```python
from build123d import *

# Parameters (mm, degrees)
F0_R      = 10.5
F0_R_2    = 9.9
F1_DEPTH  = 1.7
F2_DEPTH  = 2.8
F3_R      = 10.5
F4_DEPTH  = 1.7
F5_R      = 11
F6_DEPTH  = 8
F7_SIZE2  = 4
F7_SIZE   = 3
F8_R      = 8
F9_DEPTH  = 5
F11_D     = 18
F11_DEPTH = 10
F11_TIP   = 5.4077455712
F13_D     = 12
F14_R     = 1


with BuildPart() as f1:
    # F0 (on Top) → F1 (new body)
    with BuildSketch(Plane.XY):
        Circle(F0_R)
        Circle(F0_R_2, mode=Mode.SUBTRACT)
    extrude(amount=F1_DEPTH)

    # F0 (on Top) → F2 (join)
    with BuildSketch(Plane.XY):
        Circle(F0_R_2)
    extrude(amount=F2_DEPTH)

    # F3 (on face) → F4 (join)
    with BuildSketch(Plane.XY.offset(2.8)):
        Circle(F3_R)
    extrude(amount=F4_DEPTH)

    # F5 (on face) → F6 (join)
    with BuildSketch(Plane.XY.offset(4.5)):
        Circle(F5_R)
    extrude(amount=F6_DEPTH)

    # F7
    f7_edges = [f1.edges().sort_by_distance(p)[0] for p in [
        (-11, 0, 12.5),
    ]]
    f7_side = f1.faces().sort_by_distance((0, 0, 12.5))[0]
    chamfer(f7_edges, length=F7_SIZE, length2=F7_SIZE2, reference=f7_side)

    # F8 (on face) → F9 (join)
    with BuildSketch(Plane.XY.offset(12.5)):
        Circle(F8_R)
    extrude(amount=F9_DEPTH)

    # F11
    with Locations(Plane(origin=(0, 0, 0), x_dir=(1, 0, 0), z_dir=(0, 0, -1))):
        with Locations((0, 0)):
            Hole(F11_D / 2, depth=F11_DEPTH)
            with Locations((0, 0, -(F11_DEPTH + F11_TIP / 2))):  # 118° drill point
                Cone(0, F11_D / 2, F11_TIP, mode=Mode.SUBTRACT)

    # F13 (through all)
    with Locations(Plane.XY.offset(17.5)):
        with Locations((0, 0)):
            Hole(F13_D / 2)

    # F14
    f14_edges = [f1.edges().sort_by_distance(p)[0] for p in [
        (-8, 0, 17.5),
    ]]
    fillet(f14_edges, radius=F14_R)


solid = f1.part
```
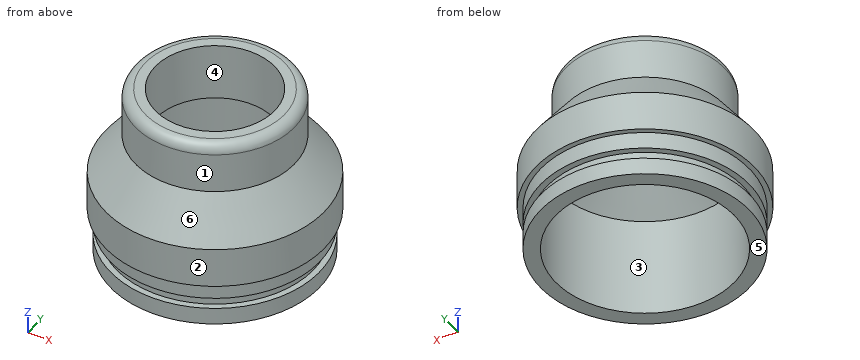
The listing builds one solid part. Answer for the finished solid, in the listing's coordinates (mm). Face numbers are marked on the shaded views. A direction names the side the tool comes from. Give positions to 0.01 mm unless a question says otherwise; leave off trailing zeros. Order: outer loops, then holes, each group sorted by start corner. A loop starts at its lowest first (then second) coordinate and runs counter-clockwise, first axis right, second up. Notation, with made-up numbers: (-34, -28.75) -> (14, -28.75) arc R26 cw to (14, 10.25) -> close; hole circle Ø1 at (12, 43.5). An arc over 180 degrees is marked (long way). One line per item, written item: value.
1) Flat-ended cylindrical pins translate along their axes: P1, Ø10, axis at y = 7.5, z = 9.5, coming from the -X side; P2, Ø1, axis at x = -3, y = -3.5, coming from the -Z side; P3, Ø3, axis at x = -6, z = 9, coming from the -Y side; P4, Ø6.5, axis at x = -4.5, y = 1, coming from the -Z side. Find the tip coordinate at first contact, or state that the pin passes through.
Reported:
P1: stops at x = -10.69
P2: passes through
P3: stops at y = -10
P4: stops at z = 10.69
2) Determine the mould class of the marked faces 3, 4, 5 and 6 for opening direction Y: pulls with the +Y half, pulls with the -Y half, needs draft (parallel to the pull), parting line crosses it, or undercut.
Reported:
face 3: undercut
face 4: undercut
face 5: needs draft
face 6: parting line crosses it
3) Find section C-C, the plane z = 2.5. Determine the outline of the cut face in (x, y), plus the area to 3 significant figures.
Reported:
outline: circle Ø19.8 at (0, 0); hole circle Ø18 at (0, 0)
area: 53.4 mm^2
4) A tool of negligible diameter and unlimited length cuts with its end or side. For the marked faces 1 and 2, from which of +Z, -Z, +X, -X, +Y, -Y can it reach the whole face along a straight path? Write none if from no direction.
Reported:
face 1: +Z
face 2: +Z, -Z
5) Find the intervals of material crossed by line 1 (Y direction, x = 0, z = 7); line 2 (Y direction, x = 0, z = 16.3); line 3 (Z direction, x = 8.75, y = -5), in increasing order.
Reported:
line 1: y = -11 to -9, 9 to 11
line 2: y = -8 to -6, 6 to 8
line 3: z = 0 to 1.7, 2.8 to 9.73
6) Find section D-D, the plane z = 9.5. Determine the outline of the cut face in (x, y), plus the area to 3 significant figures.
Reported:
outline: circle Ø20.5 at (0, 0); hole circle Ø18 at (0, 0)
area: 75.6 mm^2
